Build history of the part. All positions in model axes, mm. Face numbers are marked on the shaded views. A direction names the side the tool comes from. Round coordinates to 2 decimals unless told otherwise and drop trailing zeros. Order: outer loops, then holes, each group sorted by start corner. A loop starts at its lowest first (then second) coordinate and runs counter-clockwise, first axis right, second up. Notation, with made-up numbers: (15, 26.25) -> (56, 26.25) arc R19 ccw to (56, 58.25) -> close; hole circle Ø5 at (38, -31). An arc over 180 degrees is marked (long way). Use a Markdown table: item, result. Add a question column.
Item 1: Slice it at B-B, the plane z = 3.5. Give the cut face in (x, y).
Item 2: Pin check, flat tips, straight feed: pin 1 (0.8 mm diameter, centred on y = -0.5, z = -2.5, fed in from +X); pin 2 (0.5 mm diameter, centred on y = -0.5, z = 11, fed in from -X); pin 3 (1 mm diameter, centred on x = 7, z = 10.5, fed in from -Y). Stop position of each tip, or through.
Item 3: Slice it at C-C, the plane x = -4.5. Give the cut face in (y, z).
Item 4: Slice it at A-A, the plane y = -0.45. Give the cut face in (x, z), plus the area to 3 significant figures.
Item 5: 3-axis set-ups, long thin cutter, end or side, ignore diameter. For the marked faces 1 and 2: which of +Z, -Z, +X, -X, +Y, -Y reach the whole face in a straight line?
Item 6: Slice it at D-D, the plane z = 15. Give the cut face in (x, y), plus the area to 3 significant figures.
Item 7: Probe L1, parallel to X at y = -1.3, z = -6.5; L2, parallel to X at y = -0.8, z = 9; L3, parallel to Z at x = -2, y = -0.05. List the from-to ranges inside material, lowest first.
Item 8: Two-plate mould, pull along X, no slides. Class the marked faces 3 and 4: released by +X, released by -X, zero draft, split by the parting line, or undercut.
from build123d import *

# Parameters (mm, degrees)
F0_W     = 4.9639665522
F0_H     = 0.5
F0_W_2   = 5.0214207731
F1_DEPTH = 1
F2_DEPTH = 8.4
F4_DEPTH = 0.75


with BuildPart() as f1:
    # F0 (on Front) → F1 (new body)
    with BuildSketch(Plane.XZ):
        with BuildLine():
            Line((-5.0214207731, -9.1), (0, -9.1))
            Line((0, -9.1), (4.9639665522, -9.1))
            Line((4.9639665522, -9.1), (4.9639665522, -9.6))
            Line((4.9639665522, -9.6), (16, -9.6))
            ThreePointArc((16, -9.6), (16.7734096476, -4.8284801716), (17, 0))
            Line((17, 0), (17, 16.2837651256))
            ThreePointArc((17, 16.2837651256), (15.8919740301, 19.4226404256), (13.0589847405, 21.1703335861))
            ThreePointArc((13.0589847405, 21.1703335861), (6.5662809494, 22.1758593321), (0, 22.4))
            ThreePointArc((0, 22.4), (-6.5662809494, 22.1758593321), (-13.0589847405, 21.1703335861))
            ThreePointArc((-13.0589847405, 21.1703335861), (-15.8919740301, 19.4226404256), (-17, 16.2837651256))
            Line((-17, 16.2837651256), (-17, 0))
            ThreePointArc((-17, 0), (-16.7734096476, -4.8284801716), (-16, -9.6))
            Line((-16, -9.6), (-5.0214207731, -9.6))
            Line((-5.0214207731, -9.6), (-5.0214207731, -9.1))
        make_face()
        Polygon((5, -8), (0, -8), (-5, -8), (-5, 14), (5, 14), align=None, mode=Mode.SUBTRACT)
        with Locations((2.4819832761, -9.35)):
            Rectangle(F0_W, F0_H)
        with Locations((-2.5107103866, -9.35)):
            Rectangle(F0_W_2, F0_H)
    extrude(amount=F1_DEPTH)

    # F0 (on Front) → F2 (cut)
    with BuildSketch(Plane.XZ):
        with Locations((-2.5107103866, -9.35)):
            Rectangle(F0_W_2, F0_H)
        with Locations((2.4819832761, -9.35)):
            Rectangle(F0_W, F0_H)
    extrude(amount=F2_DEPTH, mode=Mode.SUBTRACT)

    # F3 (on face) → F4 (join)
    with BuildSketch(Plane.XZ.offset(1)):
        with BuildLine():
            Line((-13.4512646501, -9.6), (-12.4512640759, -9.6))
            Line((-12.4512640759, -9.6), (-12.4512640759, 16.2837651256))
            Line((-12.4512640759, 16.2837651256), (-15.5969633106, 19.7567832571))
            ThreePointArc((-15.5969633106, 19.7567832571), (-15.9307044856, 19.3740017261), (-16.223895747, 18.9593407121))
            Line((-16.223895747, 18.9593407121), (-13.4512646501, 15.8982095126))
            Line((-13.4512646501, 15.8982095126), (-13.4512646501, -9.6))
        make_face()
        with BuildLine():
            Line((12.4512640759, 16.2837651256), (12.4512640759, -9.6))
            Line((12.4512640759, -9.6), (13.4512646501, -9.6))
            Line((13.4512646501, -9.6), (13.4512646501, 15.8982095126))
            Line((13.4512646501, 15.8982095126), (16.223895747, 18.9593407121))
            ThreePointArc((16.223895747, 18.9593407121), (15.9307044856, 19.3740017261), (15.5969633106, 19.7567832571))
            Line((15.5969633106, 19.7567832571), (12.4512640759, 16.2837651256))
        make_face()
    extrude(amount=F4_DEPTH)


solid = f1.part
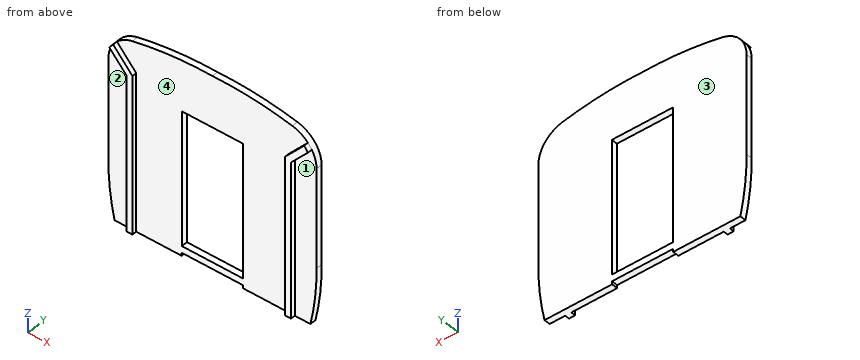
Check sheet entries:
| question | item | result |
|---|---|---|
| 1 | outline | (-17, -1) -> (-13.45, -1) -> (-13.45, -1.75) -> (-12.45, -1.75) -> (-12.45, -1) -> (-5, -1) -> (-5, 0) -> (-17, 0) -> close; (5, -1) -> (12.45, -1) -> (12.45, -1.75) -> (13.45, -1.75) -> (13.45, -1) -> (17, -1) -> (17, 0) -> (5, 0) -> close |
| 2 | pin 1 | x = 16.97 |
| 2 | pin 2 | x = -17 |
| 2 | pin 3 | y = -1 |
| 3 | outline | (-1, -9.1) -> (0, -9.1) -> (0, -8) -> (-1, -8) -> close; (-1, 14) -> (0, 14) -> (0, 22.33) -> (-1, 22.33) -> close |
| 4 | outline | (-17, 0) arc R42.5 ccw to (-16, -9.6) -> (-5.02, -9.6) -> (-5.02, -9.1) -> (4.96, -9.1) -> (4.96, -9.6) -> (16, -9.6) arc R42.5 ccw to (17, 0) -> (17, 16.28) arc R5 ccw to (13.06, 21.17) arc R55 ccw to (0, 22.4) arc R55 ccw to (-13.06, 21.17) arc R5 ccw to (-17, 16.28) -> close; hole (-5, -8) -> (5, -8) -> (5, 14) -> (-5, 14) -> close |
| 4 | area | 828 mm2 |
| 5 | face 1 | -Z, +X, -Y |
| 5 | face 2 | -Z, -X, -Y |
| 6 | outline | (-17, -1) -> (-13.45, -1) -> (-13.45, -1.75) -> (-12.45, -1.75) -> (-12.45, -1) -> (12.45, -1) -> (12.45, -1.75) -> (13.45, -1.75) -> (13.45, -1) -> (17, -1) -> (17, 0) -> (-17, 0) -> close |
| 6 | area | 35.5 mm2 |
| 7 | L1 | -13.45 to -12.45, 12.45 to 13.45 |
| 7 | L2 | -17 to -5, 5 to 17 |
| 7 | L3 | -9.1 to -8, 14 to 22.41 |
| 8 | face 3 | zero draft |
| 8 | face 4 | undercut |
